from build123d import *

# Parameters (mm, degrees)
PIN_DRAWING_W       = 0.636
PIN_DRAWING_H       = 0.636
BOSS_EXTRUDE1_DEPTH = 2.54


with BuildPart() as part:
    # pin_drawing → Boss-Extrude1 (new body)
    with BuildSketch(Plane.XY):
        Polygon((-0.014377737, 2.079116284), (-0.014377737, 0.25314904), (0.339175653, -0.107330326), (-0.014377737, -0.460883716), (-0.014377737, -2.28685096), (0.339175653, -2.647330326), (2.164719162, -2.647330326), (2.518272553, -2.293776935), (2.518272553, -0.46648), (2.164719162, -0.107330326), (2.518272553, 0.246223065), (2.518272553, 2.07352), (2.164719162, 2.432669674), (2.518272553, 2.786223065), (2.518272553, 4.61352), (2.164719162, 4.972669674), (2.518272553, 5.326223065), (2.518272553, 7.15352), (2.164719162, 7.512669674), (2.518272553, 7.866223065), (2.518272553, 9.69352), (2.164719162, 10.052669674), (2.518272553, 10.406223065), (2.518272553, 12.23352), (2.164719162, 12.592669674), (2.518272553, 12.946223065), (2.518272553, 14.77352), (2.164719162, 15.132669674), (2.518272553, 15.486223065), (2.518272553, 17.31352), (2.164719162, 17.672669674), (2.518272553, 18.026223065), (2.518272553, 19.85352), (2.164719162, 20.212669674), (2.518272553, 20.566223065), (2.518272553, 22.39352), (2.164719162, 22.752669674), (2.518272553, 23.106223065), (2.518272553, 24.93352), (2.164719162, 25.292669674), (2.518272553, 25.646223065), (2.518272553, 27.47352), (2.164719162, 27.832669674), (0.339175653, 27.832669674), (-0.014377737, 27.479116284), (-0.014377737, 25.65314904), (0.339175653, 25.292669674), (-0.014377737, 24.939116284), (-0.014377737, 23.11314904), (0.339175653, 22.752669674), (-0.014377737, 22.399116284), (-0.014377737, 20.57314904), (0.339175653, 20.212669674), (-0.014377737, 19.859116284), (-0.014377737, 18.03314904), (0.339175653, 17.672669674), (-0.014377737, 17.319116284), (-0.014377737, 15.49314904), (0.339175653, 15.132669674), (-0.014377737, 14.779116284), (-0.014377737, 12.95314904), (0.339175653, 12.592669674), (-0.014377737, 12.239116284), (-0.014377737, 10.41314904), (0.339175653, 10.052669674), (-0.014377737, 9.699116284), (-0.014377737, 7.87314904), (0.339175653, 7.512669674), (-0.014377737, 7.159116284), (-0.014377737, 5.33314904), (0.339175653, 4.972669674), (-0.014377737, 4.619116284), (-0.014377737, 2.79314904), (0.339175653, 2.432669674), align=None)
        with Locations((1.256122263, -1.357330326)):
            Rectangle(PIN_DRAWING_W, PIN_DRAWING_H, mode=Mode.SUBTRACT)
        with Locations((1.256122263, 1.182669674)):
            Rectangle(PIN_DRAWING_W, PIN_DRAWING_H, mode=Mode.SUBTRACT)
        with Locations((1.256122263, 3.722669674)):
            Rectangle(PIN_DRAWING_W, PIN_DRAWING_H, mode=Mode.SUBTRACT)
        with Locations((1.256122263, 6.262669674)):
            Rectangle(PIN_DRAWING_W, PIN_DRAWING_H, mode=Mode.SUBTRACT)
        with Locations((1.256122263, 8.802669674)):
            Rectangle(PIN_DRAWING_W, PIN_DRAWING_H, mode=Mode.SUBTRACT)
        with Locations((1.256122263, 11.342669674)):
            Rectangle(PIN_DRAWING_W, PIN_DRAWING_H, mode=Mode.SUBTRACT)
        with Locations((1.256122263, 13.882669674)):
            Rectangle(PIN_DRAWING_W, PIN_DRAWING_H, mode=Mode.SUBTRACT)
        with Locations((1.256122263, 16.422669674)):
            Rectangle(PIN_DRAWING_W, PIN_DRAWING_H, mode=Mode.SUBTRACT)
        with Locations((1.256122263, 18.962669674)):
            Rectangle(PIN_DRAWING_W, PIN_DRAWING_H, mode=Mode.SUBTRACT)
        with Locations((1.256122263, 21.502669674)):
            Rectangle(PIN_DRAWING_W, PIN_DRAWING_H, mode=Mode.SUBTRACT)
        with Locations((1.256122263, 24.042669674)):
            Rectangle(PIN_DRAWING_W, PIN_DRAWING_H, mode=Mode.SUBTRACT)
        with Locations((1.256122263, 26.582669674)):
            Rectangle(PIN_DRAWING_W, PIN_DRAWING_H, mode=Mode.SUBTRACT)
    extrude(amount=BOSS_EXTRUDE1_DEPTH)


solid = part.part
CAD build for the part. Positions are in the model's coordinates, mm. Give positions to 0.01 mm unless a question says otherwise; leave off trailing zeros. Write each loop counter-clockwise with the first axis right and the second up, starting at its lowest first coordinate (ties: lowest second). Pieces come first, ordered by that corner, then holes. Notation, with made-up numbers: (62, -2) - (76, -2) arc R23 cw to (76, 28) - close; hole circle Ø5 at (63.25, -28.5). An arc over 180 degrees is marked (long way). Answer as CSV lines item,"result".
Q1. Band-saw the part on A-A (y = 21.5). Give the cut face in (x, z).
Result set:
outline,"(-0.01, 0) - (0.94, 0) - (0.94, 2.54) - (-0.01, 2.54) - close; (1.57, 0) - (2.52, 0) - (2.52, 2.54) - (1.57, 2.54) - close"
Q2. Band-saw the part on B-B (x = 1.2). State how many separate pieces and enclosed holes the cut face has, and give its area (3 significant figures).
Result set:
separate pieces,"13"
enclosed holes,"0"
area,"58.0 mm²"
Q3. Drill centre lines: line 1 (X direction, y = 1, z = 1.7); line 2 (X direction, y = 17.5, z = 1.7); line 3 (X direction, y = 20.5, z = 0.75). Where is each one in solid material? Low to high. Write a range as from..to.
Result set:
line 1,"-0.01..0.94, 1.57..2.52"
line 2,"0.17..2.33"
line 3,"0.06..2.45"
